Answer from the drawing. Dimensions are ordinates in mm from the lowest x, y and z of the part. Coordinates: 2 decimals unless noted, no trailing zeros. Loops run counter-clockwise (first coordinate to the right, second up) from the corner with the lowest first, then second, coordinate; pieces in that order, holes last. Notation, with made-up numbers: M 16.5,49.5 L 21.5,49.5 A17 cw 21.5,72.5 Z; hole C 83.5,15 d4. An arc over 180 degrees is marked long. Put each result on its own line as item: value.
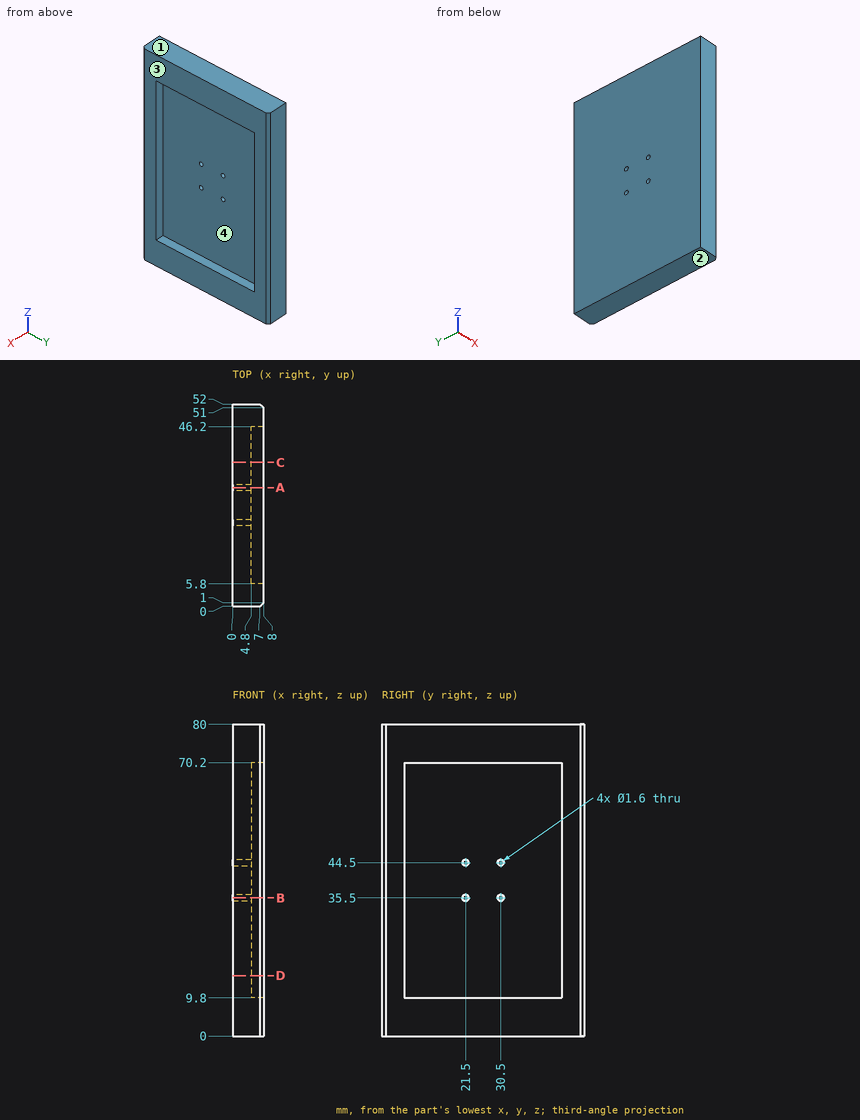
1) Given pin 1 Ø5 at (y, z) = (43, 71.5) entering from -X; pin 2 Ø2.5 at (y, z) = (21.5, 35.5) entering from +X; pin 3 Ø1 at (y, z) = (30.5, 44.5) entering from -X, each flat-ended and moving along its own axis, determine where each tip first touches the part or whether it passes through.
Answer list:
pin 1: stops at x = 0
pin 2: stops at x = 4.8
pin 3: passes through
2) Find section B-B, the plane z = 35.5. Write down the section's boundary in (x, y), plus the area to 3 significant figures.
Answer list:
outline: M 0,0 L 7,0 L 8,1 L 8,5.8 L 4.8,5.8 L 4.8,20.7 L 0,20.7 Z; M 0,22.3 L 4.8,22.3 L 4.8,29.7 L 0,29.7 Z; M 0,31.3 L 4.8,31.3 L 4.8,46.2 L 8,46.2 L 8,51 L 7,52 L 0,52 Z
area: 270 mm^2
3) Find section C-C, the plane y = 37. Write down the section's boundary in (x, z).
Answer list:
outline: M 0,0 L 8,0 L 8,9.8 L 4.8,9.8 L 4.8,70.2 L 8,70.2 L 8,80 L 0,80 Z
4) Find section A-A, the plane y = 30.5. Write down the section's boundary in (x, z), plus the area to 3 significant figures.
Answer list:
outline: M 0,0 L 8,0 L 8,9.8 L 4.8,9.8 L 4.8,34.7 L 0,34.7 Z; M 0,36.3 L 4.8,36.3 L 4.8,43.7 L 0,43.7 Z; M 0,45.3 L 4.8,45.3 L 4.8,70.2 L 8,70.2 L 8,80 L 0,80 Z
area: 431 mm^2
5) Determine the mould class of the marked faces 1, 2, 3 and 4 for opening direction Z: released by +Z, released by -Z, zero draft, split by the parting line, or undercut.
Answer list:
face 1: released by +Z
face 2: released by -Z
face 3: zero draft
face 4: undercut
6) Straight lines are drawn through the part: line 1 (Y direction, x = 2.9, z = 35.5); line 2 (Z direction, x = 7, y = 15); line 3 (Z direction, x = 3, y = 30). For each, find the intervals that lie inside material, in ascending order. Write a range as [from, to].
Answer list:
line 1: y = [0, 20.7], [22.3, 29.7], [31.3, 52]
line 2: z = [0, 9.8], [70.2, 80]
line 3: z = [0, 34.88], [36.12, 43.88], [45.12, 80]
7) Find section D-D, the plane z = 15.5. Write down the section's boundary in (x, y), plus the area to 3 significant figures.
Answer list:
outline: M 0,0 L 7,0 L 8,1 L 8,5.8 L 4.8,5.8 L 4.8,46.2 L 8,46.2 L 8,51 L 7,52 L 0,52 Z
area: 286 mm^2
